```python
from build123d import *

# Parameters (mm, degrees)
SKETCH_1_W           = 150
SKETCH_1_H           = 80
EXTRUDE_1_DEPTH      = 60
CUT_EXTRUDE_2_DEPTH  = 60
SKETCH_3_W           = 50
SKETCH_3_H           = 2
CUT_EXTRUDE_3_DEPTH  = 35
SKETCH_4_W           = 2
SKETCH_4_H           = 50
CUT_EXTRUDE_4_DEPTH  = 35
SKETCH_5_R           = 30
EXTRUDE_2_DEPTH      = 60
CUT_EXTRUDE_5_DEPTH  = 58
SKETCH_7_R           = 20
CUT_EXTRUDE_8_DEPTH  = 62
SKETCH_8_W           = 58.287497292
SKETCH_8_H           = 2
CUT_EXTRUDE_12_DEPTH = 35
SKETCH_10_W          = 2
SKETCH_10_H          = 50
EXTRUDE_6_DEPTH      = 2


with BuildPart() as part:
    # 草图1 → 凸台-拉伸1 (new body)
    with BuildSketch(Plane.XY):
        Rectangle(SKETCH_1_W, SKETCH_1_H)
    extrude(amount=EXTRUDE_1_DEPTH)

    # 草图2 → 切除-拉伸2 (cut)
    with BuildSketch(Plane.XY.offset(60)):
        Polygon((75, 0), (37.5, -40), (75, -40), align=None)
    extrude(amount=-CUT_EXTRUDE_2_DEPTH, mode=Mode.SUBTRACT)

    # 草图3 → 切除-拉伸3 (cut)
    with BuildSketch(Plane(origin=(0, 40, 0), x_dir=(1, 0, 0), z_dir=(0, 1, 0))):
        with Locations((-50, -56.5)):
            Rectangle(SKETCH_3_W, SKETCH_3_H)
        with Locations((-50, -3.5)):
            Rectangle(SKETCH_3_W, SKETCH_3_H)
        with Locations((50, -56.5)):
            Rectangle(SKETCH_3_W, SKETCH_3_H)
        with Locations((50, -3.5)):
            Rectangle(SKETCH_3_W, SKETCH_3_H)
    extrude(amount=-CUT_EXTRUDE_3_DEPTH, mode=Mode.SUBTRACT)

    # 草图4 → 切除-拉伸4 (cut)
    with BuildSketch(Plane(origin=(39.916839917, -37.422037422, 0), x_dir=(0, 0, -1), z_dir=(0.7295372041400852, -0.6839411288813299, 0))):
        with Locations((-3, 23.880944417)):
            Rectangle(SKETCH_4_W, SKETCH_4_H)
        with Locations((-57, 23.880944417)):
            Rectangle(SKETCH_4_W, SKETCH_4_H)
    extrude(amount=-CUT_EXTRUDE_4_DEPTH, mode=Mode.SUBTRACT)

    # 草图5 → 凸台-拉伸2 (add)
    with BuildSketch(Plane.XZ.offset(40)):
        with Locations(Location((-18.75, 30, 0), (0, 0, 270))):
            Circle(SKETCH_5_R)
    extrude(amount=EXTRUDE_2_DEPTH)

    # 草图6 → 切除-拉伸5 (cut)
    with BuildSketch(Plane(origin=(0, 0, 0), x_dir=(-1, 0, 0), z_dir=(0, 0, -1))):
        Polygon((73, -38), (73, 38), (-73, 38), (-73, 0.79089496), (-36.633535975, -38), align=None)
    extrude(amount=-CUT_EXTRUDE_5_DEPTH, mode=Mode.SUBTRACT)

    # 草图7 → 切除-拉伸8 (cut)
    with BuildSketch(Plane.XZ.offset(100)):
        with Locations(Location((-18.75, 30, 0), (0, 0, 270))):
            Circle(SKETCH_7_R)
    extrude(amount=-CUT_EXTRUDE_8_DEPTH, mode=Mode.SUBTRACT)

    # 草图8 → 切除-拉伸12 (cut)
    with BuildSketch(Plane(origin=(39.916839917, -37.422037422, 0), x_dir=(0, 0, -1), z_dir=(0.7295372041400852, -0.6839411288813299, 0))):
        with Locations((-33.143748646, 50.380944417)):
            Rectangle(SKETCH_8_W, SKETCH_8_H)
        with Locations((-33.143748646, -2.619055583)):
            Rectangle(SKETCH_8_W, SKETCH_8_H)
    extrude(amount=-CUT_EXTRUDE_12_DEPTH, mode=Mode.SUBTRACT)

    # 草图10 → 凸台-拉伸6 (add)
    with BuildSketch(Plane(origin=(39.916839917, -37.422037422, 0), x_dir=(0, 0, -1), z_dir=(0.7295372041400852, -0.6839411288813299, 0))):
        with Locations((-57, 23.880944417)):
            Rectangle(SKETCH_10_W, SKETCH_10_H)
        with Locations((-3, 23.880944417)):
            Rectangle(SKETCH_10_W, SKETCH_10_H)
    extrude(amount=-EXTRUDE_6_DEPTH)


solid = part.part
```
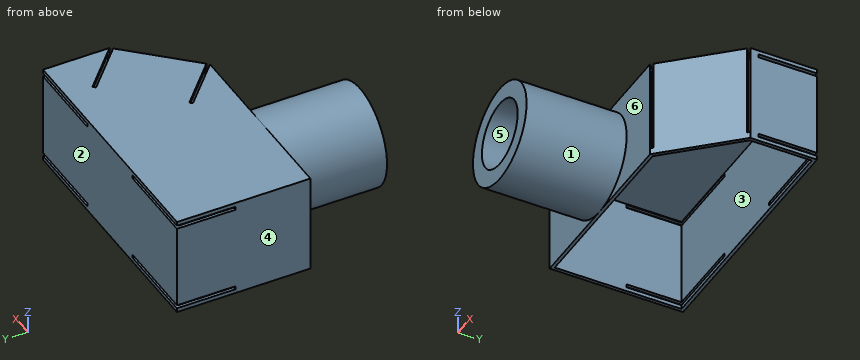
Geometry: final body of the model. Coordinates: model frame, mm. Face numbers are marked on the shaded views. A direction names the side the tool comes from. Coordinates: 2 decimals unless noted, no trailing zeros. Order: outer loops, then holes, each group sorted by start corner. A loop starts at its lowest first (then second) coordinate and runs counter-clockwise, first axis right, second up. Notation, with made-up numbers: M -5,56.5 L 52,56.5 A24 cw 52,67.5 Z; hole C 16.5,25.25 d5. An arc over 180 degrees is marked long. Answer as CSV lines item,"result".
Q1. Section D-D on y = 8. Return the cut outline in (x, z), and give its area (3 significant figures).
Answers:
outline,"M -75,0 L -73,0 L -73,2.5 L -75,2.5 Z; M -75,4.5 L -73,4.5 L -73,55.5 L -75,55.5 Z; M -75,57.5 L -73,57.5 L -73,58 L 63.67,58 L 63.67,60 L -75,60 Z; M 66.59,58 L 73,58 L 73,57.5 L 75,57.5 L 75,60 L 66.59,60 Z; M 73,0 L 75,0 L 75,2.5 L 73,2.5 Z; M 73,4.5 L 75,4.5 L 75,55.5 L 73,55.5 Z"
area,"510 mm^2"
Q2. Draft query along X for the marked faces 4, 5 and 6. Return one class per face: pulls with the +X half, pulls with the -X half, needs draft (parallel to the pull), parting line crosses it, or undercut.
Answers:
face 4,"pulls with the -X half"
face 5,"undercut"
face 6,"needs draft"
Q3. Line query: probe 1 along Y at (x, z) = (-57, 39.5); probe 2 along Y at (x, z) = (-27, 5); probe 3 along X at (y, z) = (21, 23). Output: solid intervals per line, ascending. Write a range as [from, to].
Answers:
probe 1,"y = [-40, -38], [38, 40]"
probe 2,"y = [-100, -38], [38, 40]"
probe 3,"x = [-75, -73], [73, 75]"
Q4. Section C-C on z = 31.5. Return the cut outline in (x, y).
Answers:
outline,"M -75,-40 L -48.71,-40 L -48.71,-100 L -38.69,-100 L -38.69,-38 L -73,-38 L -73,38 L 73,38 L 73,1.99 L 75,0.12 L 75,40 L -75,40 Z; M 1.19,-100 L 11.21,-100 L 11.21,-40 L 37.38,-40 L 35.24,-38 L 1.19,-38 Z; M 37.35,-37.24 L 38.81,-38.6 L 73.69,-1.4 L 72.23,-0.03 Z"
Q5. Section A-A on x = 41. Return the cut outline in (y, z).
Answers:
outline,"M -36.27,0 L -33.34,0 L -33.34,58 L 38,58 L 38,57.5 L 40,57.5 L 40,60 L -36.27,60 Z; M 38,0 L 40,0 L 40,2.5 L 38,2.5 Z; M 38,4.5 L 40,4.5 L 40,55.5 L 38,55.5 Z"
Q6. Section B-B on x = -11. Return the cut outline in (y, z), and give its area (3 significant figures).
Answers:
outline,"M -100,1.02 L -40,1.02 L -40,0 L -38,0 L -38,11.56 L -100,11.56 Z; M -100,48.44 L -38,48.44 L -38,58 L 38,58 L 38,0 L 40,0 L 40,60 L -40,60 L -40,58.98 L -100,58.98 Z"
area,"1,580 mm^2"
Q7. First-contact query: P1, Ø1, axis at y = -79.5, z = 44, coming from the +X side; P2, Ø3, axis at x = 19, z = 28, coming from the -Y side; P3, Ø5, axis at x = -12, y = -61, coming from the +Z side. Flat tips, straight axial feed; report the tip coordinate or a pass-through.
Answers:
P1,"stops at x = 8.04"
P2,"stops at y = -40"
P3,"stops at z = 59.7"
Q8. Set-up query: the marked faces 1, 2 and 3. Return all of +Z, -Z, +X, -X, +Y, -Y with unobstructed straight access to the full face (end or side cutting, diameter ignored); none if empty.
Answers:
face 1,"-Y"
face 2,"+Z, -Z, +X, -X, +Y"
face 3,"-Z"
